from build123d import *

# Parameters (mm, degrees)
F0_R     = 30
F0_R_2   = 25
F1_DEPTH = 1100
F2_R     = 30
F3_DEPTH = 8
F4_R     = 4
F4_R_2   = 2
F5_DEPTH = 1108


with BuildPart() as f1:
    # F0 (on Top) → F1 (new body)
    with BuildSketch(Plane.XY):
        Circle(F0_R)
        Circle(F0_R_2, mode=Mode.SUBTRACT)
    extrude(amount=F1_DEPTH)

    # F2 (on face) → F3 (join)
    with BuildSketch(Plane(origin=(0, 0, 0), x_dir=(1, 0, 0), z_dir=(0, 0, -1))):
        Circle(F2_R)
    extrude(amount=F3_DEPTH)

    # F4 (on face) → F5 (join)
    with BuildSketch(Plane(origin=(0, 0, -8), x_dir=(1, 0, 0), z_dir=(0, 0, -1))):
        Circle(F4_R)
        with Locations((-20, 0)):
            Circle(F4_R_2)
    extrude(amount=-F5_DEPTH)


solid = f1.part
Input: part model. Units: mm. Frame: model coordinates. A direction names the side the tool comes from. Coordinates: 2 decimals unless noted, no trailing zeros. Order: outer loops, then holes, each group sorted by start corner. A loop starts at its lowest first (then second) coordinate and runs counter-clockwise, first axis right, second up. Notation, with made-up numbers: M 2.25,58.5 L 27.25,58.5 A18 cw 27.25,63.5 Z; hole C 40.25,64.5 d2. An arc over 180 degrees is marked long. Answer in a Markdown table with one row per item.
(1) Draft query along Y for faces 1 (the flat face through (0, 0, -8)), 2 (the cylindrical face through (-29.97, -1.32, 553.76)), 3 (the flat face through (0, 5, 0)). Return one class per face: pulls with the +Y half, pulls with the -Y half, needs draft (parallel to the pull), parting line crosses it, or undercut.
Numbers:
| item | result |
|---|---|
| face 1 | needs draft |
| face 2 | parting line crosses it |
| face 3 | undercut |
(2) Section query A-A, the plane z = 462. Output: boundary loops of the cut face in (x, y).
Numbers:
| item | result |
|---|---|
| outline | C 0,0 d60; C -20,0 d4; C 0,0 d8; hole C 0,0 d50 |
(3) Access query for faces 4 (the flat face through (-7, 25, 1100)), 5 (the cylindrical face through (23.846, 7.509, 542.3)). Directions: +Z, -Z, +X, -X, +Y, -Y. A direction counts if a zero-diameter tool reaches every point of the face in a straight line with its end or side. Return the directions, or none.
Numbers:
| item | result |
|---|---|
| face 4 | +Z, +X, -X, +Y, -Y |
| face 5 | +Z |
(4) Material intervals for line 1 (Y direction, x = 0, z = 302.5); line 2 (X direction, y = 3, z = 531); line 3 (X direction, y = -9, z = 860), sorted ascending. Write a range as [from, to].
Numbers:
| item | result |
|---|---|
| line 1 | y = [-30, -25], [-4, 4], [25, 30] |
| line 2 | x = [-29.85, -24.82], [-2.65, 2.65], [24.82, 29.85] |
| line 3 | x = [-28.62, -23.32], [23.32, 28.62] |
(5) Contact query for flat-ended pins moving along their axis: pin 1 Ø2 at (x, z) = (23.5, 681.5) entering from -Y; pin 2 Ø5 at (y, z) = (3.5, 519) entering from -X; pin 3 Ø1 at (x, z) = (15, 699) entering from +Y. Output: stop coordinate, or through.
Numbers:
| item | result |
|---|---|
| pin 1 | stops at y = -19.84 |
| pin 2 | stops at x = -29.98 |
| pin 3 | stops at y = 26.26 |
